Work out the finished part from the listing and answer in its coordinate system (mm). Face numbers are marked on the shaded views. A direction names the side the tool comes from. Round coordinates to 2 decimals unless told otherwise and drop trailing zeros. Write each loop counter-clockwise with the first axis right and the second up, starting at its lowest first coordinate (ties: lowest second). Pieces come first, ordered by that corner, then holes. Notation, with made-up numbers: M 12.25,-15 L 57.25,-15 A20 ccw 57.25,-1 Z; hole C 61.25,3 d10. An arc over 180 degrees is marked long. One line per item, written item: value. Start each with the question number.
Q1. Find section B-B (x = -13.5). Write down the section's boundary in (y, z) (3 decimals).
Q2. Find section D-D (x = -11.25). Write down the section's boundary in (y, z) (3 decimals).
Q3. The mould has two halves that part along X. Classify the marked faces 1, 2 and 3: released by +X, released by -X, zero draft, split by the parting line, or undercut.
Q4. Find section C-C (y = 4). Write down the section's boundary in (x, z), and give its area (3 significant figures).
Q5. Consider probe 1 along X at (y, z) = (4.75, -5.5); probe 2 along X at (y, z) = (1.75, -3.5); probe 3 along Y at (x, z) = (-12, -4). Determine where each line is inside the solid, lowest interval first.
Q6. A tool of negligible diameter and unlimited length cuts with its end or side. For the marked faces 4 and 5, from which of +Z, -Z, +X, -X, +Y, -Y can it reach the whole face along a straight path? Write none if from no direction.
Q7. Given pin 1 Ø5 at (x, z) = (-4.78, -4.78) entering from +Y; pin 2 Ø4.5 at (x, z) = (-14.5, -6) entering from +Y; pin 3 Ø2 at (x, y) = (-13, 5) entering from -Z, each flat-ended and moving along its own axis, determine where each tip first touches the part or whether it passes through.
Q8. Find section A-A (z = -3.75). Write down the section's boundary in (x, y) (3 decimals).
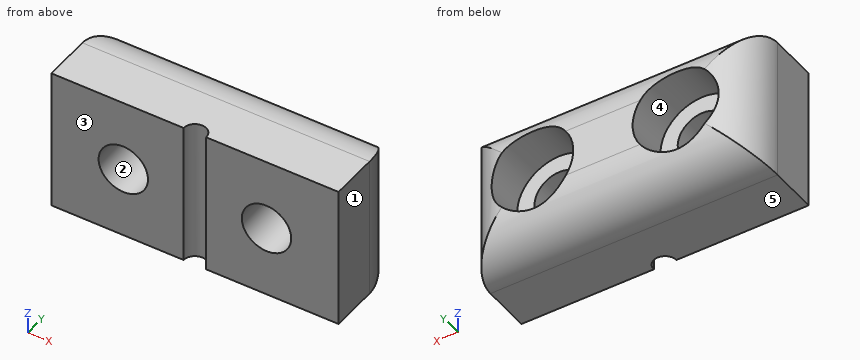
Autodesk Inventor part; units mm, degrees
ref_plane "YZ Plane" through (0, 0, 0) normal (1, 0, 0) x (0, 1, 0)
ref_plane "XZ Plane" through (0, 0, 0) normal (0, 1, 0) x (-1, 0, 0)
ref_plane "XY Plane" through (0, 0, 0) normal (0, 0, 1) x (1, 0, 0)
sketch "Sketch1" plane through (0, 0, 0) normal (0, 1, 0) x (-1, 0, 0)
  line L0 (0, 0) -> (19.05, 0)
  line L1 (19.05, 0) -> (19.05, -9.525)
  line L2 (19.05, -9.525) -> (0, -9.525)
  line L3 (0, -9.525) -> (0, 0)
  dimension "d0" = 19.05
  dimension "d1" = 9.525
extrude "Extrusion1" add sketch "Sketch1" along normal blind 6.35
sketch "Sketch2" plane through (-19.05, 0, 0) normal (0, 0, 1) x (1, 0, 0)
  line L0 (19.05, 0) -> (0, 0)
  point P0 (9.525, 0)
hole "Hole1" at (-9.525, 0, 0) direction (0, 0, -1) diameter 1.5 end through all
sketch "Sketch3" plane through (0, 6.35, 0) normal (0, 1, 0) x (1, 0, 0)
  line L0 (-19.05, 0) -> (-10.275, 0)
  line L1 (-19.05, 0) -> (-14.2748, 0)
  line L2 (-14.2748, 0) -> (-14.2748, 4.7752)
  line L3 (-14.2748, 4.7752) -> (-19.05, 4.7752)
  line L4 (-19.05, 4.7752) -> (-19.05, 0)
  line L5 (-19.05, 0) -> (0, 0)
  line L6 (0, 0) -> (-4.7752, 0)
  line L7 (-4.7752, 0) -> (-4.7752, 4.7752)
  line L8 (-4.7752, 4.7752) -> (0, 4.7752)
  line L9 (0, 4.7752) -> (0, 0)
  dimension "d11" = 4.7752
  dimension "d12" = 4.7752
  dimension "d13" = 4.7752
  dimension "d14" = 4.7752
hole "Hole2" at (-14.2748, 6.35, -4.7752) at (-4.7752, 6.35, -4.7752) direction (0, -1, 0) diameter 3.2766 end through all counterbore diameter 5.5626 counterbore depth 2.8448
sketch "Sketch4" plane through (0, 0, 0) normal (1, 0, 0) x (0, 0, -1)
  point P0 (0, 0)
fillet "Fillet1" radius 3.175 4 edges at (-9.525, 6.35, 0) (0, 6.35, -4.7625) (-9.525, 6.35, -9.525) (-19.05, 6.35, -4.7625)
properties part number "Top clamp for capillary jig - thermal seal"
The answers:
1. outline: M 0,-9.525 L 3.175,-9.525 A3.175 ccw 6.155,-7.446 L 3.505,-7.446 L 3.505,-6.219 L 0,-6.219 Z; M 0,-3.332 L 3.505,-3.332 L 3.505,-2.104 L 6.164,-2.104 A3.175 ccw 3.175,0 L 0,0 Z
2. outline: M 0,-9.525 L 3.175,-9.525 A3.175 ccw 6.35,-6.35 L 6.35,-3.175 A3.175 ccw 3.175,0 L 0,0 Z
3. face 1: released by +X
3. face 2: undercut
3. face 3: zero draft
4. outline: M -18.94,-9.42 L -0.11,-9.42 L -0.11,-0.11 L -18.94,-0.11 Z; hole C -14.27,-4.78 d5.56; hole C -4.78,-4.78 d5.56
4. area: 127 mm2
5. probe 1: -18.63 to -16.96, -11.59 to -7.46, -2.09 to -0.42
5. probe 2: -19.05 to -15.3, -13.25 to -5.8, -3.75 to 0
5. probe 3: 0 to 3.51
6. face 4: +Y
6. face 5: -Z, +X, -X, +Y, -Y
7. pin 1: y = 3.51
7. pin 2: y = 6.33
7. pin 3: z = -9.42
8. outline: M -19.05,0 L -15.553,0 L -15.553,3.505 L -16.86,3.505 L -16.86,6.193 A3.175 ccw -19.05,3.175 Z; M -12.997,0 L -10.275,0 A0.75 cw -8.775,0 L -6.053,0 L -6.053,3.505 L -7.361,3.505 L -7.361,6.35 L -11.689,6.35 L -11.689,3.505 L -12.997,3.505 Z; M -3.497,0 L 0,0 L 0,3.175 A3.175 ccw -2.19,6.193 L -2.19,3.505 L -3.497,3.505 Z
